```python
from build123d import *

# Parameters (mm, degrees)
CIRPATTERN1_COUNT = 3


with BuildPart() as part:
    # Sketch1 → Revolve1 (revolve)
    with BuildSketch(Plane(origin=(0, 0, 0), x_dir=(0, 0, -1), z_dir=(1, 0, 0))):
        Polygon((-6.7945, 0), (-11.43, 0), (-11.43, 85.725), (7.62, 85.725), (7.62, 76.2), (-6.7945, 76.2), align=None)
    revolve(axis=Axis((0, 0, 0), (0, 0, 1)))

    # Sketch8 → #10-32 Tapped Hole1 (revolve, cut)
    with BuildSketch(Plane(origin=(85.725, 0, 0), x_dir=(0, 0, -1), z_dir=(0, 1, 0))):
        Polygon((0, 0), (0, 86.937317848), (2.0193, 85.724), (2.0193, 0), align=None)
    f_10_32_tapped_hole1 = revolve(axis=Axis((92.075, 0, 0), (-1, 0, 0)), mode=Mode.SUBTRACT)

    # CirPattern1: #10-32 Tapped Hole1 ×3 about axis
    cirpattern1_axis = Axis((0, 0, 0), (0, 0, -1))
    for i in range(1, CIRPATTERN1_COUNT):
        add(f_10_32_tapped_hole1.rotate(cirpattern1_axis, i * 360 / CIRPATTERN1_COUNT), mode=Mode.SUBTRACT)


solid = part.part
```
Model file for the job. Use its own axes, mm. A direction names the side the tool comes from. Coordinates: 2 decimals unless noted, no trailing zeros. Loops run counter-clockwise (first coordinate to the right, second up) from the corner with the lowest first, then second, coordinate; pieces in that order, holes last. Notation, with made-up numbers: (2, 50.25) -> (33, 50.25) arc R34 ccw to (33, 86.25) -> close; hole circle Ø1 at (10.25, 61). An arc over 180 degrees is marked (long way). Answer as a JSON object with one key per item and string values.
Q1. Cut at B-B (z = 0). List the corners of the cut face in (x, y) (3 decimals), and give its area (3 significant figures).
Report:
{"outline": "(-44.599, -73.21) -> (-39.835, -64.958) arc R76.2 cw to (-39.835, 64.958) -> (-44.599, 73.21) arc R85.725 ccw to start; (-41.102, -75.229) arc R85.725 ccw to (85.701, -2.019) -> (76.173, -2.019) arc R76.2 cw to (-36.338, -66.978) -> close; (-41.102, 75.229) -> (-36.338, 66.978) arc R76.2 cw to (76.173, 2.019) -> (85.701, 2.019) arc R85.725 ccw to start", "area": "4,730 mm2"}
Q2. Cut at A-A (y = 0). List the corners of the cut face in (x, z) (1 decimal), and give its area (3 significant figures).
Report:
{"outline": "(-85.7, -7.6) -> (-76.2, -7.6) -> (-76.2, 6.8) -> (76.2, 6.8) -> (76.2, 2) -> (85.7, 2) -> (85.7, 11.4) -> (-85.7, 11.4) -> close; (76.2, -7.6) -> (85.7, -7.6) -> (85.7, -2) -> (76.2, -2) -> close", "area": "1,030 mm2"}
Q3. Cut at D-D (y = 22). List the corners of the cut face in (x, z).
Report:
{"outline": "(-82.85, -7.62) -> (-72.96, -7.62) -> (-72.96, 6.79) -> (72.96, 6.79) -> (72.96, -7.62) -> (82.85, -7.62) -> (82.85, 11.43) -> (-82.85, 11.43) -> close"}
Q4. Flat gauge pins, fed straight in: P1, Ø2, axis at x = 24, y = -9, coming from the -Z side; P2, Ø3, axis at y = -14, z = 4.5, coming from the -X side; P3, Ø2.5, axis at y = 0, z = 0, coming from the +X side. Where does each tip first touch, or does it go through?
Report:
{"P1": "stops at z = 6.79", "P2": "stops at x = -84.81", "P3": "stops at x = -76.19"}
Q5. Probe probe 1 along X at (y, z) = (0, -3.75) (3 decimals); probe 2 along Z at (x, y) = (-2.5, -5). List the from-to ranges inside material, lowest first.
Report:
{"probe 1": "x = -85.725 to -76.2, 76.2 to 85.725", "probe 2": "z = 6.79 to 11.43"}
Q6. 3-axis set-ups, long thin cutter, end or side, ignore diameter. For faces 1 (the cylindrical face through (-72.28, 46.09, 1.77)), 2 (the cylindrical face through (81.02, -1.7, -1.09)), 3 (the cylindrical face through (46.367, -60.47, -0.312)): which of +Z, -Z, +X, -X, +Y, -Y reach the whole face in a straight line?
Report:
{"face 1": "+Z, -Z", "face 2": "+X", "face 3": "-Z"}
Q7. Cut at C-C (x = 0). List the corners of the cut face in (y, z) (1 decimal).
Report:
{"outline": "(-85.7, -7.6) -> (-76.2, -7.6) -> (-76.2, 6.8) -> (76.2, 6.8) -> (76.2, -7.6) -> (85.7, -7.6) -> (85.7, 11.4) -> (-85.7, 11.4) -> close"}
Q8. Pull direction Z, two halves, no side cores. Call faces 4 (the cylindrical face through (-42.215, 69.176, 0.438)), 5 (the flat face through (50, -58, -7.62)), 6 (the flat face through (-1, 1, 11.43)): released by +Z, released by -Z, zero draft, split by the parting line, or undercut.
Report:
{"face 4": "undercut", "face 5": "released by -Z", "face 6": "released by +Z"}
